```python
from build123d import *

# Parameters (mm, degrees)
SZKIC1_R                    = 22.225
DODANIE_WYCI_GNI_CIE1_DEPTH = 20.65
WYTNIJ_WYCI_GNI_CIE1_REACH  = 39.607
DODANIE_WYCI_GNI_CIE2_DEPTH = 11.81
SZYK_KO_OWY1_COUNT          = 3
SZKIC4_R                    = 3.175
WYTNIJ_WYCI_GNI_CIE2_DEPTH  = 6.54


with BuildPart() as part:
    # Szkic1 → Dodanie-wyciągnięcie1 (new body)
    with BuildSketch(Plane.XY):
        with Locations(Location((0, 0, 0), (0, 0, 180))):
            Circle(SZKIC1_R)
    extrude(amount=DODANIE_WYCI_GNI_CIE1_DEPTH)

    # Szkic2 → Wytnij-wyciągnięcie1 (cut, up to next)
    with BuildSketch(Plane.XY.offset(20.65), mode=Mode.PRIVATE) as wytnij_wyci_gni_cie1_sk1:
        with BuildLine():
            Line((-2.44, 13.233874999), (2.44, 13.233874999))
            Line((2.44, 13.233874999), (2.44, 10.843874999))
            ThreePointArc((2.44, 10.843874999), (0, -11.115), (-2.44, 10.843874999))
            Line((-2.44, 10.843874999), (-2.44, 13.233874999))
        make_face()
    wytnij_wyci_gni_cie1_tool1 = extrude(wytnij_wyci_gni_cie1_sk1.sketch, amount=-WYTNIJ_WYCI_GNI_CIE1_REACH, mode=Mode.PRIVATE) & part.part
    add(wytnij_wyci_gni_cie1_tool1.solids().sort_by_distance((0, 0.327718, 20.65))[0], mode=Mode.SUBTRACT)

    # Szkic3 → Dodanie-wyciągnięcie2 (add)
    with BuildSketch(Plane.XY.offset(20.65)):
        with BuildLine():
            ThreePointArc((0, -12.5), (-2.026821276, -12.33458534), (-4, -11.842719282))
            Line((-4, -11.842719282), (-9, -20.321186604))
            ThreePointArc((-9, -20.321186604), (-4.599578933, -21.743838176), (0, -22.225))
            Line((0, -22.225), (0, -12.5))
        make_face()
        with BuildLine():
            ThreePointArc((4, -11.842719282), (2.026821276, -12.33458534), (0, -12.5))
            Line((0, -12.5), (0, -22.225))
            ThreePointArc((0, -22.225), (4.599578933, -21.743838176), (9, -20.321186604))
            Line((9, -20.321186604), (4, -11.842719282))
        make_face()
    dodanie_wyci_gni_cie2 = extrude(amount=DODANIE_WYCI_GNI_CIE2_DEPTH)

    # Szyk kołowy1: Dodanie-wyciągnięcie2 ×3 about axis
    szyk_ko_owy1_axis = Axis((0, 0, 0), (0, 0, 1))
    for i in range(1, SZYK_KO_OWY1_COUNT):
        add(dodanie_wyci_gni_cie2.rotate(szyk_ko_owy1_axis, i * 360 / SZYK_KO_OWY1_COUNT))

    # Szkic4 → Wytnij-wyciągnięcie2 (cut)
    with BuildSketch(Plane(origin=(0, 22.225, 0), x_dir=(1, 0, 0), z_dir=(0, 1, 0))):
        with Locations(Location((0, -6, 0), (0, 0, 270))):
            Circle(SZKIC4_R)
    extrude(amount=-WYTNIJ_WYCI_GNI_CIE2_DEPTH, mode=Mode.SUBTRACT)


solid = part.part
```
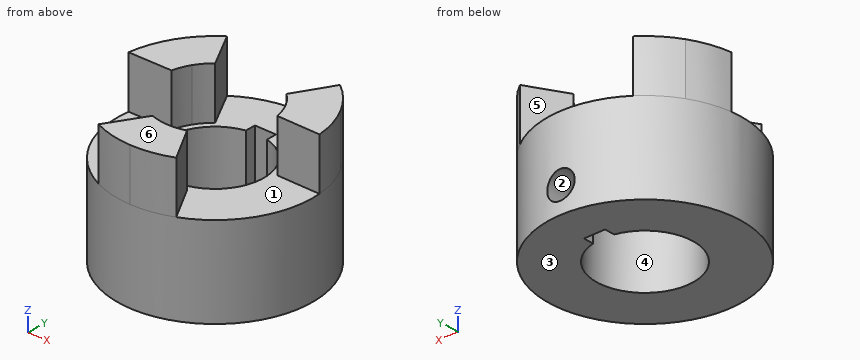
Could you check a few things on this model? Use its own coordinates, in mm. Face numbers are marked on the shaded views. A direction names the side the tool comes from. Round coordinates to 2 decimals unless told otherwise and drop trailing zeros. Write each loop counter-clockwise with the first axis right and the second up, starting at its lowest first coordinate (ties: lowest second). Pieces come first, ordered by that corner, then holes. Notation, with made-up numbers: M 81,1.5 L 133,1.5 A12 ccw 133,6.5 Z; hole C 72,76.25 d2. An arc over 180 degrees is marked long. Write each question's results on one line, items separated by ' | '. Start each with the question number.
1. Imagine slicing it at A-A on y = 0. List the corners of the cut face in (x, z) for me (3 decimals).
2. Imagine slicing it at D-D on z = 6. List the corners of the cut face in (x, y) for me (3 decimals), and give its area (3 significant figures).
3. Thinking about a two-plate mould opening in Y: for the marked faces 4, 5 and 6, which applies, +Y half, -Y half, draft (parallel to the pull), parting line (faces both ways), or undercut?
4. Imagine slicing it at C-C on x = -6. List the corners of the cut face in (y, z) for me.
5. Imagine slicing it at B-B on z = 28.5. Count the separate pieces of the cut face and the enclosed holes in it, and give its area (3 significant figures).
6. I need wall thicknesses on L1, parallel to Z at x = 0, y = 18.25 (3 decimals); L2, parallel to Z at x = 14, y = -11; L3, parallel to Y at x = 0, z = 8 (3 decimals). Which ranges of each line are inside material? Lowest first, please. Write a range as from..to.
7. On a 3-axis mill with a long thin cutter (end or side, diameter ignored), from which of +Z, -Z, +X, -X, +Y, -Y can I reach the whole of each face in a straight line? I mean the marked faces 1, 2 and 3. Say none if no direction works.
8. I'm going to push flat-ended pins straight in: pin 1 Ø1.9 at (y, z) = (11.5, 10.5) entering from +X; pin 2 Ø12 at (y, z) = (13, 19) entering from -X; pin 3 Ø3 at (x, z) = (-11.5, 4) entering from +Y. Where does each tip first touch, or does it pass through?
Result sheet:
1) outline: M -22.225,0 L -11.115,0 L -11.115,20.65 L -22.225,20.65 Z; M 11.115,0 L 22.225,0 L 22.225,20.65 L 11.115,20.65 Z
2) outline: M -3.175,15.685 L -3.175,21.997 A22.225 ccw long 3.175,21.997 L 3.175,15.685 Z; hole M -2.44,10.844 A11.115 ccw long 2.44,10.844 L 2.44,13.234 L -2.44,13.234 Z | area: 1,110 mm^2
3) face 4: undercut | face 5: +Y half | face 6: draft
4) outline: M -21.4,0 L -9.36,0 L -9.36,20.65 L -15.23,20.65 L -15.23,32.46 L -21.4,32.46 Z; M 9.36,0 L 21.4,0 L 21.4,20.65 L 9.36,20.65 Z
5) separate pieces: 3 | enclosed holes: 0 | area: 389 mm^2
6) L1: z = 0..2.825, 9.175..20.65 | L2: z = 0..20.65 | L3: y = -22.225..-11.115, 13.234..15.685
7) face 1: +Z | face 2: +Y | face 3: -Z, +X, -X, +Y, -Y
8) pin 1: stops at x = 19.56 | pin 2: stops at x = -21.09 | pin 3: stops at y = 19.85
